Can you work these out from the model? Positions are in its coordinate system, mm. A direction names the side the tool comes from. Give positions to 0.01 mm unless a question says otherwise; leave off trailing zeros. Order: outer loops, then holes, each group sorted by start corner. A loop starts at its lowest first (then second) coordinate and runs counter-clockwise, first axis right, second up. Notation, with made-up numbers: (73, 11.25) - (98, 11.25) arc R26 ccw to (98, 45.25) - close; hole circle Ø6 at (81, 30.5). An arc over 180 degrees is marked (long way). Return JSON: item names as keys, results as strings.
```python
from build123d import *

# Parameters (mm, degrees)
SKETCH2_W           = 40
SKETCH2_H           = 40
BOSS_EXTRUDE1_DEPTH = 3
FILLET1_R           = 5
CUT_EXTRUDE1_REACH  = 59.446
SKETCH4_R           = 12.5
FILLET2_R           = 5
FILLET3_R           = 2
FILLET4_R           = 0.5


with BuildPart() as part:
    # Sketch2 → Boss-Extrude1 (new body)
    with BuildSketch(Plane(origin=(0, 0, 0), x_dir=(1, 0, 0), z_dir=(0, 1, 0))):
        Rectangle(SKETCH2_W, SKETCH2_H)
    extrude(amount=BOSS_EXTRUDE1_DEPTH)

    # Sketch3 → Revolve1 (revolve)
    with BuildSketch(Plane.XY, mode=Mode.PRIVATE) as revolve1_sk:
        Polygon((-15, 3), (-5, 50), (-2.5, 50), (-12.5, 3), align=None)
    revolve(revolve1_sk.sketch.rotate(Axis((0, -2.5, 0), (0, 1, 0)), 270), axis=Axis((0, -2.5, 0), (0, 1, 0)))

    # Fillet1
    fillet1_edges = [part.edges().sort_by_distance(p)[0] for p in [
        (20, 1.5, 20),
        (-20, 1.5, 20),
        (-20, 1.5, -20),
        (20, 1.5, -20),
    ]]
    fillet(fillet1_edges, radius=FILLET1_R)

    # Sketch4 → Cut-Extrude1 (cut, up to next)
    with BuildSketch(Plane.XZ, mode=Mode.PRIVATE) as cut_extrude1_sk1:
        with Locations(Location((0, 0, 0), (0, 0, 270))):
            Circle(SKETCH4_R)
    cut_extrude1_tool1 = extrude(cut_extrude1_sk1.sketch, amount=-CUT_EXTRUDE1_REACH, mode=Mode.PRIVATE) & part.part
    add(cut_extrude1_tool1.solids().sort_by_distance((0, 0, 0))[0], mode=Mode.SUBTRACT)

    # Fillet2
    fillet2_edges = [part.edges().sort_by_distance(p)[0] for p in [
        (0, 3, 12.5),
    ]]
    fillet(fillet2_edges, radius=FILLET2_R)

    # Fillet3
    fillet3_edges = [part.edges().sort_by_distance(p)[0] for p in [
        (0, 3, 15),
    ]]
    fillet(fillet3_edges, radius=FILLET3_R)

    # Fillet4
    fillet4_edges = [part.edges().sort_by_distance(p)[0] for p in [
        (0, 0, 12.5),
    ]]
    fillet(fillet4_edges, radius=FILLET4_R)


solid = part.part
```
1. Suppose I cut it at B-B (y = 38). List the corners of the cut face in (x, z) for me.
Checks:
{"outline": "circle Ø15.11 at (0, 0); hole circle Ø10.11 at (0, 0)"}
2. Suppose I cut it at A-A (y = 43.5). List the corners of the cut face in (x, z) for me, plus the area to 3 significant figures.
Checks:
{"outline": "circle Ø12.77 at (0, 0); hole circle Ø7.77 at (0, 0)", "area": "80.6 mm^2"}
3. On a 3-axis mill with a long thin cutter (end or side, diameter ignored), from which of +Z, -Z, +X, -X, +Y, -Y can I reach the whole of each face in a straight line? I mean faces 5 (the face through (3.755, 1.473, -11.923)), 6 (the face through (-19, 2, 18)), 7 (the face through (-18, 3, 0)). Say none if no direction works.
Checks:
{"face 5": "-Y", "face 6": "+Z, -X, +Y, -Y", "face 7": "+Y"}
4. For pin 1 Ø2 at (y, z) = (8.5, -10.5) entering from +X; pin 2 Ø10 at (x, y) = (-4.5, 10) entering from -Z; pin 3 Ø8 at (x, y) = (1.5, 29.5) entering from -Z; pin 4 Ø6 at (x, y) = (-15, 30) entering from +Z, each with a flat end and sliding along its axis, tell me the tip position at first contact or that it passes through.
Checks:
{"pin 1": "x = 10.09", "pin 2": "z = -14.29", "pin 3": "z = -10.17", "pin 4": "through"}
5. If I drill on L1, parallel to Z at x = 0, y = 1.45; L2, parallel to Y at x = 17.5, z = 6, over which ranges is the centre line in solid material (lowest first)? Write a range as [from, to].
Checks:
{"L1": "[-20, -12.5], [12.5, 20]", "L2": "[0, 3]"}
6. Thinking about a two-plate mould opening in X: for faces 1 (the face through (-20, 1, 0)), 2 (the face through (18, 2, 19)), 3 (the face through (2.88, 26.43, -6.94)), 4 (the face through (0, 1, 20)), which applies, +X half, -X half, draft (parallel to the pull), parting line (faces both ways), or undercut?
Checks:
{"face 1": "-X half", "face 2": "+X half", "face 3": "undercut", "face 4": "draft"}
